For this review, take the finished solid that the model builds, in its own axes (mm). Round coordinates to 2 decimals unless told otherwise and drop trailing zeros. Write each loop counter-clockwise with the first axis right and the second up, starting at its lowest first coordinate (ties: lowest second). Pieces come first, ordered by that corner, then holes.
Autodesk Inventor part; units mm, degrees
ref_plane "YZ Plane" through (0, 0, 0) normal (1, 0, 0) x (0, 1, 0)
ref_plane "XZ Plane" through (0, 0, 0) normal (0, 1, 0) x (-1, 0, 0)
ref_plane "XY Plane" through (0, 0, 0) normal (0, 0, 1) x (1, 0, 0)
sketch "Sketch1" plane through (0, 0, 0) normal (0, 1, 0) x (-1, 0, 0)
  circle A0 centre (0, 0) radius 37.5
  circle A1 centre (0, 0) radius 14.5
  line L0 (0, 0) -> (23.813, 0)
  circle A2 centre (23.813, 0) radius 2.56
  circle A3 centre (11.9065, 20.6227) radius 2.56
  circle A4 centre (-11.9065, 20.6227) radius 2.56
  circle A5 centre (-23.813, 0) radius 2.56
  circle A6 centre (-11.9065, -20.6227) radius 2.56
  circle A7 centre (11.9065, -20.6227) radius 2.56
  dimension "d0" = 75
  dimension "d1" = 29
  dimension "d2" = 23.813
  dimension "d3" = 5.12
  dimension "d6" = 360
extrude "Extrusion1" add sketch "Sketch1" along normal blind 10.16
properties part number "driving system S4"
(1) We need section C-C, the plane z = -13.5. Give the boundary of the cut face in (x, y).
Geometry check:
outline: (-34.99, 0) - (-5.29, 0) - (-5.29, 10.16) - (-34.99, 10.16) - close; (5.29, 0) - (34.99, 0) - (34.99, 10.16) - (5.29, 10.16) - close
(2) For line 1 along Z through (x, y) = (13, 3); line 2 along X through (y, z) = (5.25, 21); line 3 along X through (y, z) = (8, 19), list the stretches that pass through material, from the lowest coordinate up.
Geometry check:
line 1: z = -35.17 to -22.94, -18.31 to -6.42, 6.42 to 18.31, 22.94 to 35.17
line 2: x = -31.07 to -14.44, -9.37 to 9.37, 14.44 to 31.07
line 3: x = -32.33 to -13.89, -9.93 to 9.93, 13.89 to 32.33
(3) We need section B-B, the plane z = 0. Give the boundary of the cut face in (x, y), and give its area (3 significant figures).
Geometry check:
outline: (-37.5, 0) - (-26.37, 0) - (-26.37, 10.16) - (-37.5, 10.16) - close; (-21.25, 0) - (-14.5, 0) - (-14.5, 10.16) - (-21.25, 10.16) - close; (14.5, 0) - (21.25, 0) - (21.25, 10.16) - (14.5, 10.16) - close; (26.37, 0) - (37.5, 0) - (37.5, 10.16) - (26.37, 10.16) - close
area: 363 mm2
(4) We need section A-A, the plane x = 0. Give the boundary of the cut face in (y, z).
Geometry check:
outline: (0, -37.5) - (10.16, -37.5) - (10.16, -14.5) - (0, -14.5) - close; (0, 14.5) - (10.16, 14.5) - (10.16, 37.5) - (0, 37.5) - close
(5) Mouldability with a two-part tool opening along Z and no side actions: class faces 1 (the face through (-9.875, 5.009, -19.065)), 2 (the face through (1, 10.16, -16)), 3 (the face through (13.938, 5.009, -19.065)), 4 (the face through (4.88, 5.01, -37.18)) as pulls with the +Z half, pulls with the -Z half, needs draft (parallel to the pull), parting line crosses it, or undercut.
Geometry check:
face 1: undercut
face 2: needs draft
face 3: undercut
face 4: parting line crosses it
(6) We need section D-D, the plane x = 12. Give the boundary of the cut face in (y, z).
Geometry check:
outline: (0, -35.53) - (10.16, -35.53) - (10.16, -23.18) - (0, -23.18) - close; (0, -18.06) - (10.16, -18.06) - (10.16, -8.14) - (0, -8.14) - close; (0, 8.14) - (10.16, 8.14) - (10.16, 18.06) - (0, 18.06) - close; (0, 23.18) - (10.16, 23.18) - (10.16, 35.53) - (0, 35.53) - close
(7) For pin 1 Ø4 at (y, z) = (3, 29.5) entering from -X; pin 2 Ø2 at (x, y) = (-8, 6) entering from +Z; pin 3 Ø6 at (y, z) = (7.5, 28) entering from -X; pin 4 Ø4.5 at (x, z) = (-23.813, 0) entering from -Y, all flat-tipped, find the tip position at first contact; note any pin that passes through.
Geometry check:
pin 1: stops at x = -25.5
pin 2: stops at z = 36.84
pin 3: stops at x = -27.95
pin 4: passes through
